Drawing for the job (mm, zero at the part's lowest x, y, z). A direction names the side the tool comes from. Give positions to 0.01 mm unless a question says otherwise; leave off trailing zeros. Order: outer loops, then holes, each group sorted by start corner. A loop starts at its lowest first (then second) coordinate and runs counter-clockwise, first axis right, second up. Notation, with made-up numbers: (23.5, -6.5) - (59.5, -6.5) arc R18 ccw to (59.5, 23.5) - close; hole circle Ø2 at (-20.75, 74.25). An arc over 180 degrees is marked (long way). One line per item, written item: value.
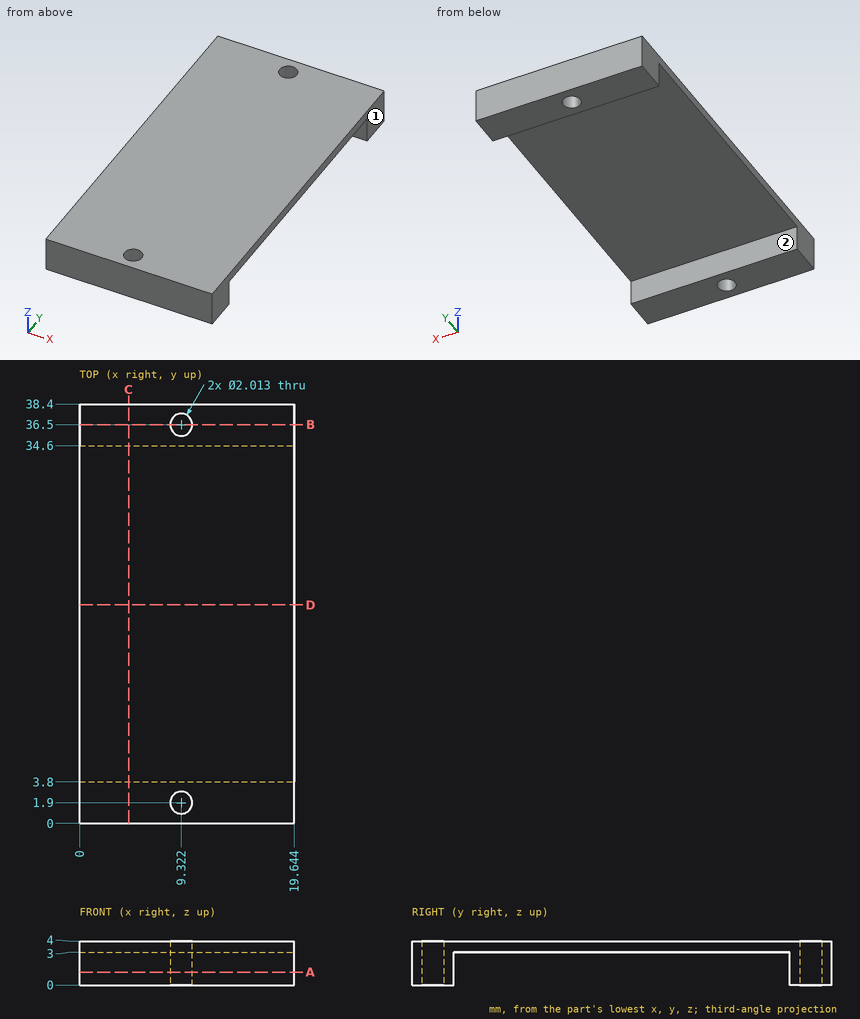
(1) Slice it at B-B, the plane y = 36.5. Give the cut face in (x, z), and give its area (3 significant figures).
Completed:
outline: (0, 0) - (8.32, 0) - (8.32, 4) - (0, 4) - close; (10.33, 0) - (19.64, 0) - (19.64, 4) - (10.33, 4) - close
area: 70.5 mm²
(2) Slice it at A-A, the plane z = 1.2. Give the cut face in (x, y).
Completed:
outline: (0, 0) - (19.64, 0) - (19.64, 3.8) - (0, 3.8) - close; (0, 34.6) - (19.64, 34.6) - (19.64, 38.4) - (0, 38.4) - close; hole circle Ø2.01 at (9.32, 1.9); hole circle Ø2.01 at (9.32, 36.5)
(3) Slice it at C-C, the plane x = 4.5. Give the cut face in (y, z), and give its area (3 significant figures).
Completed:
outline: (0, 0) - (3.8, 0) - (3.8, 3) - (34.6, 3) - (34.6, 0) - (38.4, 0) - (38.4, 4) - (0, 4) - close
area: 61.2 mm²
(4) 3-axis set-ups, long thin cutter, end or side, ignore diameter. For the marked faces 1 and 2: which of +Z, -Z, +X, -X, +Y, -Y reach the whole face in a straight line?
Completed:
face 1: +Z, -Z, +X, +Y, -Y
face 2: -Z, +X, -X
(5) Drill centre lines: line 1 (Y direction, x = 5.25, z = 0.2); line 2 (Y direction, x = 9.25, z = 0.5); line 3 (Y direction, x = 10, z = 3.1) (1 decimal). Where is each one in solid material? Low to high.
Completed:
line 1: 0 to 3.8, 34.6 to 38.4
line 2: 0 to 0.9, 2.9 to 3.8, 34.6 to 35.5, 37.5 to 38.4
line 3: 0 to 1.2, 2.6 to 35.8, 37.2 to 38.4
(6) Slice it at D-D, the plane y = 20. Give the cut face in (x, z).
Completed:
outline: (0, 3) - (19.64, 3) - (19.64, 4) - (0, 4) - close
(7) Pin check, flat tip, straight feed: P1, Ø10, axis at x = 8, y = 25, coming from the -Z side. Stop position of the tip, or through.
Completed:
P1: z = 3
